Part model, mm, in its own coordinate system. A direction names the side the tool comes from. Give positions to 0.01 mm unless a question says otherwise; leave off trailing zeros. Write each loop counter-clockwise with the first axis right and the second up, starting at its lowest first coordinate (ties: lowest second). Pieces come first, ordered by that corner, then holes. Notation, with made-up numbers: (76, 45) - (124, 45) arc R17 ccw to (124, 64) - close; hole circle Ø10 at (39.25, 20.5). An arc over 180 degrees is marked (long way). Answer in a Markdown table with one row per item. Add a question column.
1. Band-saw the part on B-B on x = 632. Write the cut outline in (y, z) (3 decimals), plus the area to 3 significant figures.
2. Band-saw the part on A-A on x = 395.5. Write the cut outline in (y, z) (3 decimals).
3. Which spindle directions (+Z, -Z, +X, -X, +Y, -Y) get a long thin tool onto all of the face, cutting with end or side? Do faces 1 (the flat face through (338, -3.175, 27)), 2 (the flat face through (338, -19, 0)). Say none if no direction does.
4. Drop flat-ended pins along their axis: pin 1 Ø10 at (x, y) = (219.075, -38.1) entering from +Z (3 decimals); pin 2 Ø12.5 at (x, y) = (482.6, -9.525) entering from -Z; pin 3 Ø12 at (x, z) = (548, 35) entering from -Y (3 decimals); pin 4 Ø2.5 at (x, z) = (82.5, 2.5) entering from -Y. Give the stop position or say it passes through.
5. Probe line 1 along X through (y, z) = (-38.1, 1.6); line 2 along Z through (x, y) = (12.7, -0.9) (3 decimals); line 3 along X through (y, z) = (-2.5, 38.1) (3 decimals). List the from-to ranges inside material, lowest first.
Autodesk Inventor part; units mm, degrees
ref_plane "YZ Plane" through (0, 0, 0) normal (1, 0, 0) x (0, 1, 0)
ref_plane "XZ Plane" through (0, 0, 0) normal (0, 1, 0) x (-1, 0, 0)
ref_plane "XY Plane" through (0, 0, 0) normal (0, 0, 1) x (1, 0, 0)
sketch "Sketch1" plane through (0, 0, 0) normal (1, 0, 0) x (0, 1, 0)
  line L0 (0, 0) -> (-3.175, 0)
  line L1 (-3.175, 0) -> (-3.175, 50.8)
  line L2 (-3.175, 50.8) -> (0, 50.8)
  line L3 (0, 50.8) -> (0, 0)
  line L4 (0, 0) -> (-50.8, 0)
  line L5 (-50.8, 0) -> (-50.8, 3.175)
  line L6 (-50.8, 3.175) -> (0, 3.175)
  line L7 (0, 3.175) -> (0, 0)
  dimension "d0" = 3.175
  dimension "d1" = 50.8
  dimension "d2" = 50.8
  dimension "d3" = 3.175
extrude "Extrusion1" add sketch "Sketch1" along normal blind 685.8
sketch "Sketch2" plane through (0, -50.8, 3.175) normal (0, 0, 1) x (1, 0, 0)
  line L0 (0, 47.625) -> (0, 0)
  line L1 (0, 0) -> (685.8, 0)
  point P0 (0, 50.8)
  point P1 (206.375, 12.7)
  point P2 (479.425, 12.7)
  point P3 (219.075, 12.7)
  point P4 (466.725, 12.7)
  dimension "d9" = 12.7
  dimension "d11" = 12.7
  dimension "d117" = 12.7
  dimension "d118" = 12.7
  dimension "d121" = 12.7
  dimension "d122" = 12.7
  dimension "d130" = 206.375
  dimension "d131" = 247.65
sketch "Sketch3" plane through (0, 0, 50.8) normal (0, 1, 0) x (1, 0, 0)
  line L0 (0, 50.8) -> (0, 0)
  line L1 (0, 0) -> (685.8, 0)
  line L2 (685.8, 50.8) -> (685.8, 0)
  line L3 (0, 50.8) -> (685.8, 50.8)
  point P0 (12.7, 12.7)
  point P1 (12.7, 38.1)
  point P2 (317.5, 19.05)
  point P3 (368.3, 19.05)
  point P4 (673.1, 12.7)
  point P5 (673.1, 38.1)
  dimension "d19" = 12.7
  dimension "d20" = 12.7
  dimension "d21" = 12.7
  dimension "d22" = 12.7
  dimension "d23" = 19.05
  dimension "d24" = 19.05
  dimension "d25" = 12.7
  dimension "d26" = 12.7
  dimension "d27" = 12.7
  dimension "d28" = 12.7
  dimension "d29" = 317.5
  dimension "d30" = 317.5
hole "Hole2" at (12.7, 0, 38.1) at (12.7, 0, 12.7) at (317.5, 0, 31.75) at (368.3, 0, 31.75) at (673.1, 0, 38.1) at (673.1, 0, 12.7) direction (0, -1, 0) diameter 6.35 end through all
sketch "Sketch4" plane through (0, 0, 50.8) normal (0, 1, 0) x (1, 0, 0)
  line L0 (0, 50.8) -> (0, 0)
  line L1 (685.8, 50.8) -> (685.8, 0)
  line L2 (0, 50.8) -> (685.8, 50.8)
  point P0 (101.6, 38.1)
  point P1 (254, 38.1)
  point P2 (431.8, 38.1)
  point P3 (584.2, 38.1)
  dimension "d38" = 101.6
  dimension "d39" = 254
  dimension "d40" = 254
  dimension "d41" = 101.6
  dimension "d42" = 12.7
  dimension "d43" = 12.7
  dimension "d44" = 12.7
  dimension "d45" = 12.7
hole "Hole3" at (101.6, 0, 12.7) at (254, 0, 12.7) at (431.8, 0, 12.7) at (584.2, 0, 12.7) direction (0, -1, 0) diameter 4.7625 end through all
sketch "Sketch6" plane through (0, -50.8, 0) normal (0, 0, -1) x (-1, 0, 0)
  line L0 (0, 0) -> (0, 50.8)
  line L1 (-685.8, 0) -> (-685.8, 50.8)
  line L2 (-685.8, 0) -> (-533.4, 0)
  line L3 (-533.4, 0) -> (-533.4, 25.4)
  line L4 (-533.4, 25.4) -> (-685.8, 25.4)
  line L5 (-685.8, 25.4) -> (-685.8, 0)
  line L6 (0, 0) -> (-152.4, 0)
  line L7 (-152.4, 0) -> (-152.4, 25.4)
  line L8 (-152.4, 25.4) -> (0, 25.4)
  line L9 (0, 25.4) -> (0, 0)
  line L10 (-685.8, 47.625) -> (-663.575, 25.4)
  line L11 (-685.8, 47.625) -> (-654.3691, 47.625) construction
  line L12 (-663.575, 25.4) -> (-685.8, 25.4)
  line L13 (-685.8, 25.4) -> (-685.8, 47.625)
  line L14 (0, 47.625) -> (-22.225, 25.4)
  line L15 (0, 47.625) -> (31.4309, 47.625) construction
  line L16 (-22.225, 25.4) -> (0, 25.4)
  line L17 (0, 25.4) -> (0, 47.625)
  line L18 (0, 47.625) -> (-685.8, 47.625)
  dimension "d65" = 152.4
  dimension "d66" = 25.4
  dimension "d67" = 152.4
  dimension "d68" = 25.4
  dimension "d69" = 45
  dimension "d70" = 135
extrude "Extrusion3" cut sketch "Sketch6" against normal blind 25.4
chamfer "Chamfer1" distance 3.175 angle 45 2 edges at (533.4, -50.8, 1.5875) (152.4, -50.8, 1.5875)
sketch "Sketch8" plane through (685.8, 0, 0) normal (0, 0, -1) x (-1, 0, 0)
  line L0 (685.8, 0) -> (0, 0)
  line L1 (0, -3.175) -> (0, 0)
  point P0 (101.6, -12.7)
  point P1 (254, -12.7)
  point P2 (431.8, -12.7)
  point P3 (584.2, -12.7)
  dimension "d91" = 12.7
  dimension "d92" = 12.7
  dimension "d93" = 12.7
  dimension "d94" = 12.7
  dimension "d95" = 101.6
  dimension "d96" = 254
  dimension "d97" = 431.8
  dimension "d98" = 584.2
hole "Hole5" at (584.2, -12.7, 0) at (431.8, -12.7, 0) at (254, -12.7, 0) at (101.6, -12.7, 0) direction (0, 0, 1) diameter 4.7625 end through all
sketch "Sketch9" plane through (0, -3.175, 3.175) normal (0, 0, 1) x (1, 0, 0)
  line L0 (0, 0) -> (685.8, 0)
  line L1 (0, 3.175) -> (0, 0)
  line L2 (685.8, 0) -> (685.8, 3.175)
  point P0 (203.2, -6.35)
  point P1 (482.6, -6.35)
  dimension "d106" = 203.2
  dimension "d107" = 6.35
  dimension "d108" = 6.35
  dimension "d109" = 203.2
hole "Hole6" at (203.2, -9.525, 3.175) at (482.6, -9.525, 3.175) direction (0, 0, -1) diameter 9.525 depth 25.4 tip angle 118
hole "Hole7" at (206.375, -38.1, 3.175) at (479.425, -38.1, 3.175) at (219.075, -38.1, 3.175) at (466.725, -38.1, 3.175) direction (0, 0, -1) diameter 6.35 depth 25.4 tip angle 118
properties part number "2x2 angle rail support" material "Aluminum 6061"
Values:
| question | item | result |
|---|---|---|
| 1 | outline | (-25.4, 0) - (0, 0) - (0, 50.8) - (-3.175, 50.8) - (-3.175, 3.175) - (-25.4, 3.175) - close |
| 1 | area | 232 mm² |
| 2 | outline | (-50.8, 0) - (0, 0) - (0, 50.8) - (-3.175, 50.8) - (-3.175, 3.175) - (-50.8, 3.175) - close |
| 3 | face 1 | +Z, +X, -X, -Y |
| 3 | face 2 | -Z, +X, -X, +Y, -Y |
| 4 | pin 1 | stops at z = 3.175 |
| 4 | pin 2 | stops at z = 0 |
| 4 | pin 3 | stops at y = -3.175 |
| 4 | pin 4 | stops at y = -25.4 |
| 5 | line 1 | x = 152.4 to 203.2, 209.55 to 215.9, 222.25 to 463.55, 469.9 to 476.25, 482.6 to 533.4 |
| 5 | line 2 | z = 0 to 9.525, 15.875 to 34.925, 41.275 to 50.8 |
| 5 | line 3 | x = 0 to 9.525, 15.875 to 669.925, 676.275 to 685.8 |
